Can you work these out from the model? Positions are in its coordinate system, mm. A direction names the side the tool comes from. Coordinates: 2 decimals unless noted, no trailing zeros. Order: outer loops, then holes, each group sorted by start corner. A loop starts at its lowest first (then second) coordinate and runs counter-clockwise, first axis right, second up. Notation, with made-up numbers: (-9.75, 67.5) - (-5.75, 67.5) arc R25 ccw to (-5.75, 97.5) - close; hole circle Ø3 at (48, 2.25). An arc over 180 degrees is marked (long way). Use a Markdown table: item, result. Add a question column.
(1) I want a section at A-A (z = 3.5). List the corners of the cut face in (x, y) for me.
(2) On a 3-axis mill with a long thin cutter (end or side, diameter ignored), from which of +Z, -Z, +X, -X, +Y, -Y can I reach the whole of each face in a straight line? I mean faces 1 (the flat face through (2, 138.356, 13)), 2 (the flat face through (-36, 161, 0)), 3 (the flat face through (-25.054, 70, 13)). Say none if no direction works.
(3) I want a section at B-B (x = -49). List the corners of the cut face in (y, z) for me, and give its area (3 significant figures).
(4) If I drill on L1, parallel to X at y = 236, z = 18.5; L2, parallel to Y at x = -58.5, z = 3.25; L3, parallel to X at y = 76, z = 1.5, over which ranges is the centre line in solid material (lowest first)? Write a range as [from, to].
(5) I want a section at C-C (y = 179). List the corners of the cut face in (x, z) for me, and give its area (3 significant figures).
(6) For pin 1 Ø7.5 at (y, z) = (69.5, 15.5) entering from -X; pin 2 Ø4 at (x, z) = (1.5, 17.5) entering from +Y; pin 3 Ø1.5 at (y, z) = (190.5, 17) entering from +X; pin 4 Ø12.5 at (x, z) = (-58, 13.5) entering from -Y, each with a flat end and sliding along its axis, tell me the tip position at first contact or that it passes through.
```python
from build123d import *

# Parameters (mm, degrees)
F0_W     = 25.0537917018
F0_H     = 55.8406859636
F1_DEPTH = 25.4


with BuildPart() as f1:
    # F0 (on Top) → F1 (new body)
    with BuildSketch(Plane.XY):
        Polygon((0, 138.3560597897), (0, 82.515373826), (-25.0537917018, 82.515373826), (-25.0537917018, 57.3403835297), (3.8365423679, 57.3403835297), (3.8365423679, 138.3560597897), align=None)
        with Locations((-12.5268958509, 110.4357168078)):
            Rectangle(F0_W, F0_H)
        Polygon((-74.49362427, 82.515373826), (-25.0537917018, 82.515373826), (-25.0537917018, 138.3560597897), (0, 138.3560597897), (0, 261.0465288162), (-74.49362427, 261.0465288162), align=None)
    extrude(amount=F1_DEPTH)


solid = f1.part
```
Answers follow:
| question | item | result |
|---|---|---|
| 1 | outline | (-74.49, 82.52) - (-25.05, 82.52) - (-25.05, 57.34) - (3.84, 57.34) - (3.84, 138.36) - (0, 138.36) - (0, 261.05) - (-74.49, 261.05) - close |
| 2 | face 1 | +Z, -Z, +X, +Y |
| 2 | face 2 | -Z, +X, -X, +Y, -Y |
| 2 | face 3 | +Z, -Z, -X, -Y |
| 3 | outline | (82.52, 0) - (261.05, 0) - (261.05, 25.4) - (82.52, 25.4) - close |
| 3 | area | 4,530 mm² |
| 4 | L1 | x = [-74.49, 0] |
| 4 | L2 | y = [82.52, 261.05] |
| 4 | L3 | x = [-25.05, 3.84] |
| 5 | outline | (-74.49, 0) - (0, 0) - (0, 25.4) - (-74.49, 25.4) - close |
| 5 | area | 1,890 mm² |
| 6 | pin 1 | stops at x = -25.05 |
| 6 | pin 2 | stops at y = 261.05 |
| 6 | pin 3 | stops at x = 0 |
| 6 | pin 4 | stops at y = 82.52 |
